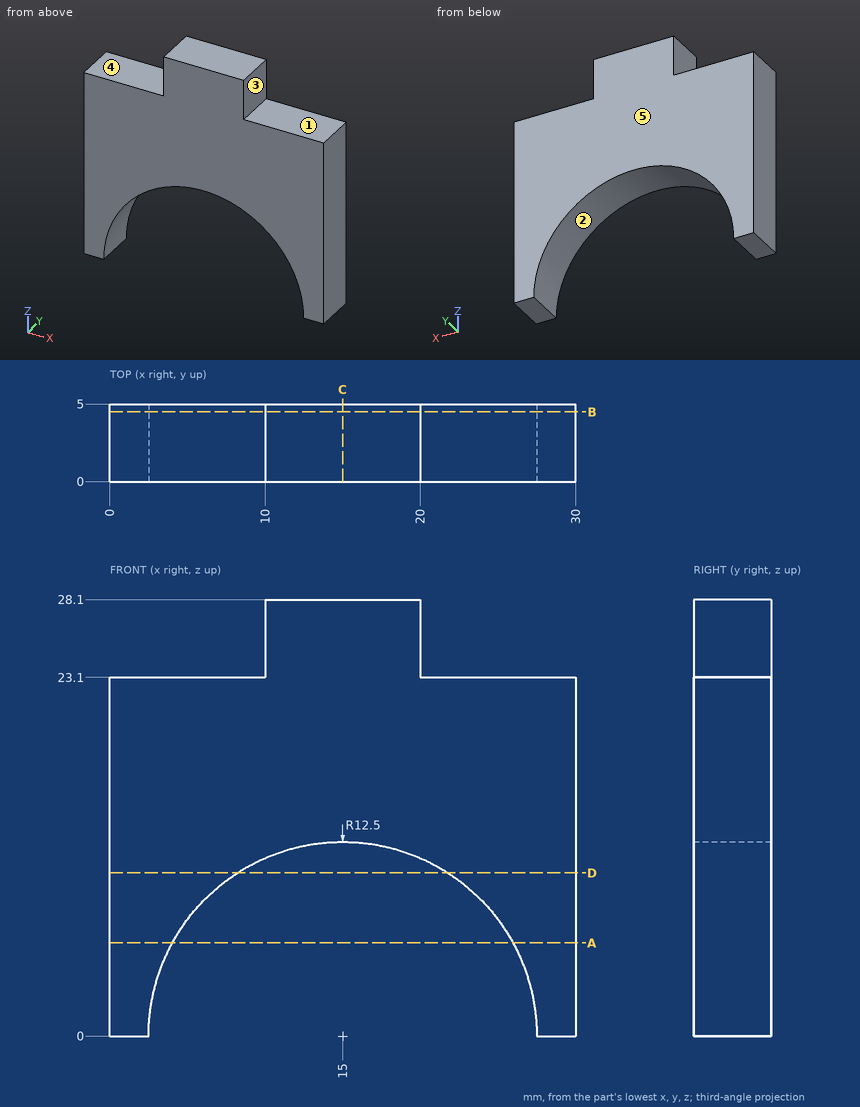
Input: dimensioned drawing with shaded views. Units: mm. Origin: part minimum x, y, z. A direction names the side the tool comes from. Give positions to 0.01 mm unless a question says otherwise; leave off trailing zeros. Write each loop counter-clockwise with the first axis right and the second up, starting at its lowest first coordinate (ties: lowest second). Pieces come first, ordered by that corner, then holes.
1. Pull-direction query (X, two-part tool) for the marked faces 1, 2 and 3; classes: +X half, -X half, draft (parallel to the pull), parting line (faces both ways), or undercut.
2. First-contact query: pin 1 (1.5 mm diameter, centred on x = 22.5, y = 3, fed in from -Z); pin 2 (1 mm diameter, centred on x = 19, y = 4, fed in from -Z); pin 3 (1 mm diameter, centred on y = 4.5, z = 13, fed in from -X); pin 4 (1.5 mm diameter, centred on y = 2.5, z = 26, fed in from -X). Flat tips, straight axial feed; report the tip coordinate or a pass-through.
3. Section query D-D (z = 10.5). Return the cut outline in (x, y).
4. Section query A-A (z = 6). Return the cut outline in (x, y).
5. Access query for the marked faces 4 and 5. Directions: +Z, -Z, +X, -X, +Y, -Y. A direction counts if a zero-diameter tool reaches every point of the face in a straight line with its end or side. Return the directions, or none.
6. Material intervals for line 1 along X through (y, z) = (3.2, 8.5); line 2 along X through (y, z) = (2.5, 26); line 3 along X through (y, z) = (4.7, 3.5), sorted ascending.
7. Section query C-C (x = 15). Return the cut outline in (y, z).
8. Section query B-B (y = 4.5). Return the cut outline in (x, z).
Output values:
1. face 1: draft
1. face 2: undercut
1. face 3: +X half
2. pin 1: stops at z = 9.39
2. pin 2: stops at z = 11.66
2. pin 3: stops at x = 0
2. pin 4: stops at x = 10
3. outline: (0, 0) - (8.22, 0) - (8.22, 5) - (0, 5) - close; (21.78, 0) - (30, 0) - (30, 5) - (21.78, 5) - close
4. outline: (0, 0) - (4.03, 0) - (4.03, 5) - (0, 5) - close; (25.97, 0) - (30, 0) - (30, 5) - (25.97, 5) - close
5. face 4: +Z, -X, +Y, -Y
5. face 5: +Z, -Z, +X, -X, +Y
6. line 1: x = 0 to 5.83, 24.17 to 30
6. line 2: x = 10 to 20
6. line 3: x = 0 to 3, 27 to 30
7. outline: (0, 12.5) - (5, 12.5) - (5, 28.1) - (0, 28.1) - close
8. outline: (0, 0) - (2.5, 0) arc R12.5 cw to (27.5, 0) - (30, 0) - (30, 23.1) - (20, 23.1) - (20, 28.1) - (10, 28.1) - (10, 23.1) - (0, 23.1) - close
